```python
from build123d import *

# Parameters (mm, degrees)
SKETCH1_W           = 60
SKETCH1_H           = 93
BOSS_EXTRUDE1_DEPTH = 4
SKETCH3_R           = 1.65
CUT_EXTRUDE1_DEPTH  = 4
SKETCH5_W           = 60
SKETCH5_H           = 4
BOSS_EXTRUDE2_DEPTH = 11
SKETCH6_W           = 123.5
SKETCH6_H           = 4
BOSS_EXTRUDE3_DEPTH = 87.5
SKETCH7_R           = 1.65
CUT_EXTRUDE2_DEPTH  = 87.5
SKETCH10_R          = 1.65
CUT_EXTRUDE3_DEPTH  = 10
SKETCH11_W          = 98.5
SKETCH11_H          = 89
BOSS_EXTRUDE4_DEPTH = 25
SKETCH13_W          = 98.5
SKETCH13_H          = 89
CUT_EXTRUDE5_DEPTH  = 8
CUT_EXTRUDE7_DEPTH  = 20
SKETCH15_W          = 71.5
SKETCH15_H          = 17
BOSS_EXTRUDE6_DEPTH = 45
CUT_EXTRUDE9_DEPTH  = 45
SKETCH17_W          = 25
SKETCH17_H          = 60
BOSS_EXTRUDE7_DEPTH = 15


with BuildPart() as part:
    # Sketch1 → Boss-Extrude1 (new body)
    with BuildSketch(Plane.XY):
        with Locations((30, -46.5)):
            Rectangle(SKETCH1_W, SKETCH1_H)
    extrude(amount=-BOSS_EXTRUDE1_DEPTH)

    # Sketch3 → Cut-Extrude1 (cut)
    with BuildSketch(Plane.XY):
        with Locations((4, -8)):
            Circle(SKETCH3_R)
        with Locations((56, -8)):
            Circle(SKETCH3_R)
        with Locations((4, -89)):
            Circle(SKETCH3_R)
        with Locations((56, -89)):
            Circle(SKETCH3_R)
    extrude(amount=-CUT_EXTRUDE1_DEPTH, mode=Mode.SUBTRACT)

    # Sketch5 → Boss-Extrude2 (add)
    with BuildSketch(Plane(origin=(0, 0, -4), x_dir=(-1, 0, 0), z_dir=(0, 0, -1))):
        with Locations((-30, -2)):
            Rectangle(SKETCH5_W, SKETCH5_H)
    extrude(amount=BOSS_EXTRUDE2_DEPTH)

    # Sketch6 → Boss-Extrude3 (add)
    with BuildSketch(Plane(origin=(0, 0, -15), x_dir=(-1, 0, 0), z_dir=(0, 0, -1))):
        with Locations((1.75, -2)):
            Rectangle(SKETCH6_W, SKETCH6_H)
    extrude(amount=BOSS_EXTRUDE3_DEPTH)

    # Sketch7 → Cut-Extrude2 (cut)
    with BuildSketch(Plane(origin=(0, 0, 0), x_dir=(1, 0, 0), z_dir=(0, 1, 0))):
        with Locations((-59.5, 98.5)):
            Circle(SKETCH7_R)
        with Locations((-36.5, 98.5)):
            Circle(SKETCH7_R)
        with Locations((-59.5, 58.5)):
            Circle(SKETCH7_R)
        with Locations((-36.5, 58.5)):
            Circle(SKETCH7_R)
    extrude(amount=-CUT_EXTRUDE2_DEPTH, mode=Mode.SUBTRACT)

    # Sketch10 → Cut-Extrude3 (cut)
    with BuildSketch(Plane(origin=(0, 0, 0), x_dir=(1, 0, 0), z_dir=(0, 1, 0))):
        with Locations((29.5, 83.25)):
            Circle(SKETCH10_R)
        with Locations((29.5, 56.75)):
            Circle(SKETCH10_R)
    extrude(amount=-CUT_EXTRUDE3_DEPTH, mode=Mode.SUBTRACT)

    # Sketch11 → Boss-Extrude4 (add)
    with BuildSketch(Plane(origin=(0, 0, 0), x_dir=(0, 0, -1), z_dir=(1, 0, 0))):
        with Locations((53.25, -48.5)):
            Rectangle(SKETCH11_W, SKETCH11_H)
    extrude(amount=BOSS_EXTRUDE4_DEPTH)

    # Sketch13 → Cut-Extrude5 (cut)
    with BuildSketch(Plane.ZY):
        with Locations((-53.25, -48.5)):
            Rectangle(SKETCH13_W, SKETCH13_H)
    extrude(amount=-CUT_EXTRUDE5_DEPTH, mode=Mode.SUBTRACT)

    # Sketch14 → Cut-Extrude7 (cut)
    with BuildSketch(Plane.ZY.offset(-8)):
        Polygon((-102.5, -4), (-102.5, -93), (-4, -93), align=None)
    extrude(amount=-CUT_EXTRUDE7_DEPTH, mode=Mode.SUBTRACT)

    # Sketch15 → Boss-Extrude6 (add)
    with BuildSketch(Plane.XZ.offset(4)):
        with Locations((-27.75, -42)):
            Rectangle(SKETCH15_W, SKETCH15_H)
    extrude(amount=BOSS_EXTRUDE6_DEPTH)

    # Sketch16 → Cut-Extrude9 (cut)
    with BuildSketch(Plane(origin=(0, 0, -50.5), x_dir=(-1, 0, 0), z_dir=(0, 0, -1))):
        Polygon((63.5, -4), (-8, -49), (63.5, -49), align=None)
    extrude(amount=-CUT_EXTRUDE9_DEPTH, mode=Mode.SUBTRACT)

    # Sketch17 → Boss-Extrude7 (add)
    with BuildSketch(Plane.XZ.offset(4)):
        with Locations((47.5, -72.5)):
            Rectangle(SKETCH17_W, SKETCH17_H)
    extrude(amount=BOSS_EXTRUDE7_DEPTH)


solid = part.part
```
The model under review builds one solid part; all positions refer to its coordinate system, in mm. A direction names the side the tool comes from. Round coordinates to 2 decimals unless told otherwise and drop trailing zeros. Write each loop counter-clockwise with the first axis right and the second up, starting at its lowest first coordinate (ties: lowest second). Pieces come first, ordered by that corner, then holes. Notation, with made-up numbers: (-2, 79.5) - (28, 79.5) arc R17 cw to (28, 107.5) - close; hole circle Ø2 at (61, 0.5). An arc over 180 degrees is marked (long way). Answer as CSV lines item,"result". Start each with the question number.
(1) For faces 5 (the flat face through (8, -28, -32)), 6 (the flat face through (47, -19, -72)), 7 (the flat face through (42, -48, -4)), list the 3-axis set-ups (+Z, -Z, +X, -X, +Y, -Y) from which the entire face can be reached by the end or side of a thin tool; tool diameter is ignored.
(2) For pin 1 Ø3 at (x, y) = (4, -8) entering from +Z; pin 2 Ø16.5 at (y, z) = (-31.5, -9.5) entering from -X; pin 3 Ø4 at (x, z) = (29.5, -83.25) entering from -Y, all flat-tipped, find the tip position at first contact; note any pin that passes through.
(3) We need section D-D on z = -83.25. State the section outline as (x, y) points.
(4) We need section C-C on x = 46.5. State the section outline as (y, z) points.
(5) To check wall thickness, follow line 1 (Y direction, x = 4, z = -2); line 2 (Z direction, x = -59.5, y = -1.75); line 3 (X direction, y = -2.3, z = -98.5). State the ranges of each line that lie inside material, in increasing order.
(6) Draft analysis for pull direction X (two halves, no side actions). For faces 1 (the flat face through (-28.25, -26.185, -42.119)), 2 (the flat face through (-12, -16, -50.5)), 3 (the cylindrical face through (54.35, -7.93, -1.97)), 4 (the flat face through (35, -11, -73)), state which applies: pulls with the +X half, pulls with the -X half, needs draft (parallel to the pull), parting line crosses it, or undercut.
(7) We need section A-A on x = 29.5. State the section outline as (y, z) points, plus the area to 3 significant figures.
(8) We need section B-B on y = -89. State the section outline as (x, z) points.
Worked answers:
1,face 5,"-X, -Y"
1,face 6,"-Z, +X, -Y"
1,face 7,"+X, -Y"
2,pin 1,"z = -33.5"
2,pin 2,"x = 0"
2,pin 3,"y = -4"
3,outline,"(-63.5, -4) - (8, -4) - (8, -21.39) - (25, -21.39) - (25, -4) - (27.85, -4) - (27.85, 0) - (-63.5, 0) - close; (31.15, -4) - (35, -4) - (35, -19) - (60, -19) - (60, 0) - (31.15, 0) - close"
4,outline,"(-93, -4) - (-4, -4) - (-4, -42.5) - (-19, -42.5) - (-19, -102.5) - (0, -102.5) - (0, 0) - (-93, 0) - close"
5,line 1,"-93 to -90.65, -87.35 to -9.65, -6.35 to 0"
5,line 2,"-102.5 to -100.15, -96.85 to -60.15, -56.85 to -15"
5,line 3,"-63.5 to -61.15, -57.85 to -38.15, -34.85 to 60"
6,face 1,"pulls with the -X half"
6,face 2,"needs draft"
6,face 3,"undercut"
6,face 4,"undercut"
7,outline,"(-93, -4) - (-4, -4) - (-4, -55.1) - (0, -55.1) - (0, 0) - (-93, 0) - close; (-4, -102.5) - (0, -102.5) - (0, -84.9) - (-4, -84.9) - close; (-4, -81.6) - (0, -81.6) - (0, -58.4) - (-4, -58.4) - close"
7,area,"740 mm²"
8,outline,"(0, -4) - (2.35, -4) - (2.35, 0) - (0, 0) - close; (5.65, -4) - (8, -4) - (8, -8.43) - (25, -8.43) - (25, -4) - (54.35, -4) - (54.35, 0) - (5.65, 0) - close; (57.65, -4) - (60, -4) - (60, 0) - (57.65, 0) - close"
